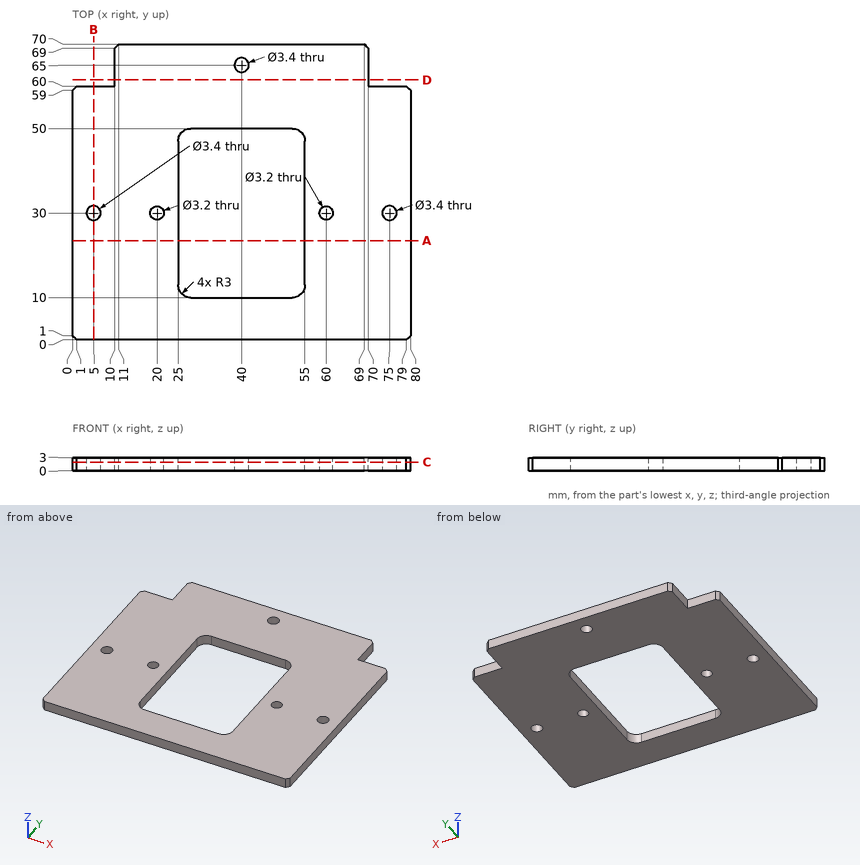
Input: dimensioned drawing with shaded views. Units: mm. Origin: part minimum x, y, z. Give positions to 0.01 mm unless a question says otherwise; leave off trailing zeros. Loops run counter-clockwise (first coordinate to the right, second up) from the corner with the lowest first, then second, coordinate; pieces in that order, holes last. Notation, with made-up numbers: (84, -31.75) -> (130, -31.75) arc R25 ccw to (130, 0.25) -> close; hole circle Ø6 at (65.25, -34.5). An arc over 180 degrees is marked (long way). Return JSON: item names as keys, results as strings.
Item 1: Section A-A, the plane y = 23.5. Output: boundary loops of the cut face in (x, z).
Filled in:
{"outline": "(0, 0) -> (25, 0) -> (25, 3) -> (0, 3) -> close; (55, 0) -> (80, 0) -> (80, 3) -> (55, 3) -> close"}
Item 2: Section B-B, the plane x = 5. Output: boundary loops of the cut face in (y, z), plus the area to 3 significant figures.
Filled in:
{"outline": "(0, 0) -> (28.3, 0) -> (28.3, 3) -> (0, 3) -> close; (31.7, 0) -> (60, 0) -> (60, 3) -> (31.7, 3) -> close", "area": "170 mm^2"}
Item 3: Section C-C, the plane z = 2. Output: boundary loops of the cut face in (x, y).
Filled in:
{"outline": "(0, 1) -> (1, 0) -> (79, 0) -> (80, 1) -> (80, 59) -> (79, 60) -> (70, 60) -> (70, 69) -> (69, 70) -> (11, 70) -> (10, 69) -> (10, 60) -> (1, 60) -> (0, 59) -> close; hole circle Ø3.4 at (5, 30); hole circle Ø3.2 at (20, 30); hole (25, 13) arc R3 ccw to (28, 10) -> (52, 10) arc R3 ccw to (55, 13) -> (55, 47) arc R3 ccw to (52, 50) -> (28, 50) arc R3 ccw to (25, 47) -> close; hole circle Ø3.4 at (40, 65); hole circle Ø3.2 at (60, 30); hole circle Ø3.4 at (75, 30)"}
Item 4: Line query: line 1 (Y direction, x = 40, z = 2.3); line 2 (X direction, y = 14.5, z = 0.65); line 3 (Y direction, x = 60, z = 1.55). Output: solid intervals per line, ascending.
Filled in:
{"line 1": "0 to 10, 50 to 63.3, 66.7 to 70", "line 2": "0 to 25, 55 to 80", "line 3": "0 to 28.4, 31.6 to 70"}
Item 5: Section D-D, the plane y = 61.5. Output: boundary loops of the cut face in (x, z).
Filled in:
{"outline": "(10, 0) -> (70, 0) -> (70, 3) -> (10, 3) -> close"}
Item 6: Pin query (flat end, axial travel): P1, Ø3, axis at x = 60, y = 30, coming from the -Z side; P2, Ø5.5, axis at x = 75, y = 30, coming from the +Z side; P3, Ø0.9, axis at y = 66.5, z = 1, coming from the +X side; P4, Ø0.9, axis at x = 5, z = 2, coming from the +Y side. Return the tip coordinate at first contact, or that it passes through.
Filled in:
{"P1": "through", "P2": "z = 3", "P3": "x = 70", "P4": "y = 60"}
